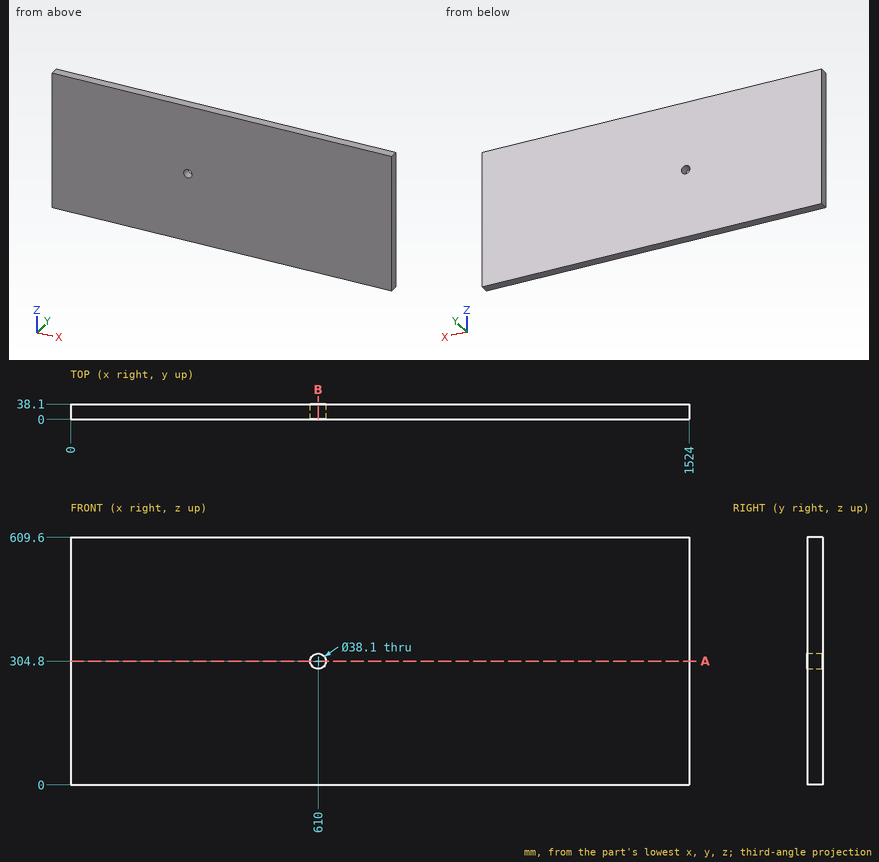
Study the drawing (mm; zero at the part's minimum x, y, z) and answer. Round coordinates to 2 decimals unless told otherwise and drop trailing zeros. Loops run counter-clockwise (first coordinate to the right, second up) from the corner with the lowest first, then second, coordinate; pieces in that order, holes last. Notation, with made-up numbers: (-21, -5) -> (-12, -5) arc R25 cw to (-12, 19) -> close; hole circle Ø2 at (-17, 83.5). An arc over 180 degrees is marked (long way). Write each question's results on one line, items separated by ' | '. Start each with the question number.
1. Find the intervals of material crossed by probe 1 along X at (y, z) = (27, 304.8); probe 2 along Z at (x, y) = (610, 25); probe 3 along X at (y, z) = (25.5, 322), in increasing order. Write a range as from..to.
2. Section B-B (x = 610) is taken. Determine the outline of the cut face in (y, z).
3. Section A-A (z = 304.8) is taken. Determine the outline of the cut face in (x, y).
Evaluation:
1) probe 1: x = 0..590.95, 629.05..1524 | probe 2: z = 0..285.75, 323.85..609.6 | probe 3: x = 0..601.81, 618.19..1524
2) outline: (0, 0) -> (38.1, 0) -> (38.1, 285.75) -> (0, 285.75) -> close; (0, 323.85) -> (38.1, 323.85) -> (38.1, 609.6) -> (0, 609.6) -> close
3) outline: (0, 0) -> (590.95, 0) -> (590.95, 38.1) -> (0, 38.1) -> close; (629.05, 0) -> (1524, 0) -> (1524, 38.1) -> (629.05, 38.1) -> close
